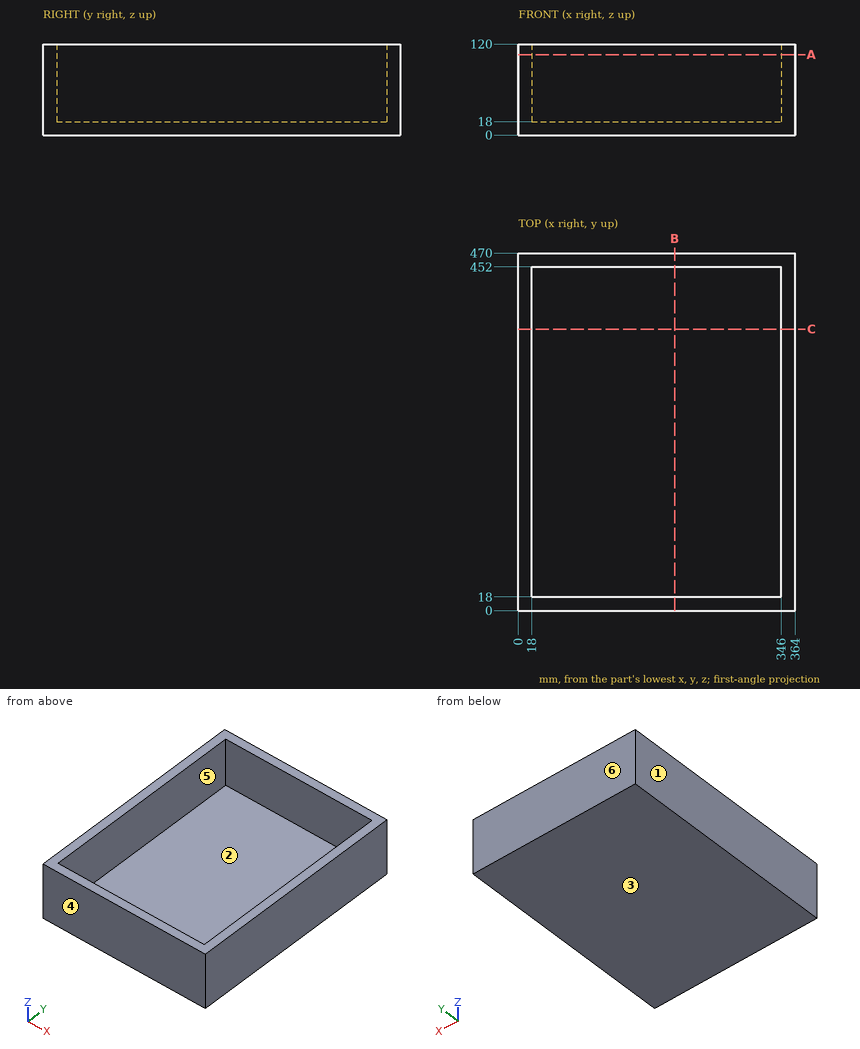
Check sheet for the drawn part. Datum: minimum x, y, z corner. Units: mm. A direction names the side the tool comes from. Give positions to 0.01 mm unless a question says otherwise; leave off trailing zeros. Loops run counter-clockwise (first coordinate to the right, second up) from the corner with the lowest first, then second, coordinate; pieces in that order, holes last. Notation, with made-up numbers: M 24.5,-34.5 L 67.5,-34.5 A15 ccw 67.5,-15.5 Z; hole C 5,-39 d1. An arc over 180 degrees is marked long. Return JSON: item names as keys, results as strings.
1) Material ranges on L1, parallel to Y at x = 255.5, z = 57; L2, parallel to X at y = 439.5, z = 62; L3, parallel to Z at x = 265.5, y = 438, recorded low to high. Write a range as [from, to].
Findings:
{"L1": "y = [0, 18], [452, 470]", "L2": "x = [0, 18], [346, 364]", "L3": "z = [0, 18]"}
2) Section check A-A, the plane z = 106. Enter the section's corners in (x, y).
Findings:
{"outline": "M 0,0 L 364,0 L 364,470 L 0,470 Z; hole M 18,18 L 346,18 L 346,452 L 18,452 Z"}
3) Mould release check, pull along Y, two halves, no side actions. Record for the marked faces 3, 4, 5 and 6: released by +Y, released by -Y, zero draft, split by the parting line, or undercut.
Findings:
{"face 3": "zero draft", "face 4": "released by -Y", "face 5": "undercut", "face 6": "released by +Y"}
4) Gauge pin test, flat ends, axial feed: P1, Ø1.5, axis at y = 191, z = 13, coming from the -X side; P2, Ø6, axis at x = 156.5, y = 48, coming from the +Z side. Record the tip position at first contact, or that the pin passes through.
Findings:
{"P1": "stops at x = 0", "P2": "stops at z = 18"}
5) Tool access check on the marked faces 1 and 2. Record the directions out of +Z, -Z, +X, -X, +Y, -Y that give a thin tool (end or side, any length) a straight path to the whole face; none if there is none.
Findings:
{"face 1": "+Z, -Z, -X, +Y, -Y", "face 2": "+Z"}
6) Section check C-C, the plane y = 370. Enter the section's corners in (x, z).
Findings:
{"outline": "M 0,0 L 364,0 L 364,120 L 346,120 L 346,18 L 18,18 L 18,120 L 0,120 Z"}
7) Section check B-B, the plane x = 205.5. Enter the section's corners in (y, z).
Findings:
{"outline": "M 0,0 L 470,0 L 470,120 L 452,120 L 452,18 L 18,18 L 18,120 L 0,120 Z"}
